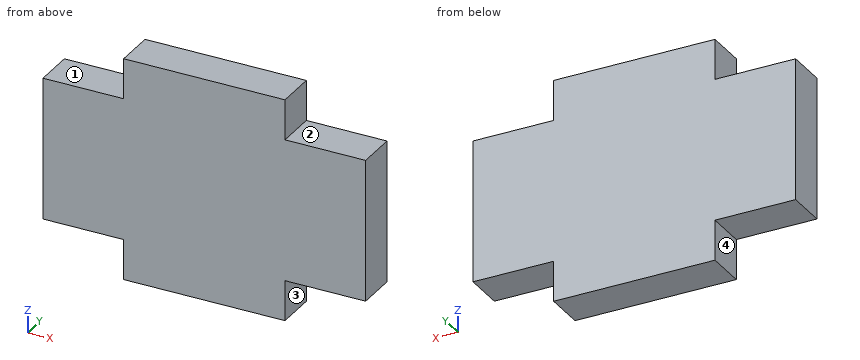
```python
from build123d import *

# Parameters (mm, degrees)
SKETCH1_W           = 12.7
SKETCH1_H           = 3.175
SKETCH1_W_2         = 6.35
BOSS_EXTRUDE1_DEPTH = 3.175


with BuildPart() as part:
    # Sketch1 → Boss-Extrude1 (new body)
    with BuildSketch(Plane(origin=(0, 0, 0), x_dir=(1, 0, 0), z_dir=(0, 1, 0))):
        Polygon((0, 11.176), (0, 0), (6.35, 0), (19.05, 0), (25.4, 0), (25.4, 11.176), (19.05, 11.176), (12.7, 11.176), (6.35, 11.176), align=None)
        with Locations((12.7, -1.5875)):
            Rectangle(SKETCH1_W, SKETCH1_H)
        with Locations((15.875, 12.7635)):
            Rectangle(SKETCH1_W_2, SKETCH1_H)
        with Locations((9.525, 12.7635)):
            Rectangle(SKETCH1_W_2, SKETCH1_H)
    extrude(amount=BOSS_EXTRUDE1_DEPTH)


solid = part.part
```
Geometry check sheet. Reference: the model listing, model coordinates, mm. Face numbers are marked on the shaded views. A direction names the side the tool comes from. Round coordinates to 2 decimals unless told otherwise and drop trailing zeros. Loops run counter-clockwise (first coordinate to the right, second up) from the corner with the lowest first, then second, coordinate; pieces in that order, holes last. Notation, with made-up numbers: (17.25, -22.75) - (41.25, -22.75) arc R29 cw to (41.25, 4.25) - close; hole circle Ø7 at (31.25, 16). An arc over 180 degrees is marked (long way). Write each question's results on one line, items separated by ' | '. Start each with the question number.
Q1. Cross-section at C-C on z = 2. Enter the section's corners in (x, y) (3 decimals), and give its area (3 significant figures).
Q2. Cross-section at A-A on y = 0.5. Enter the section's corners in (x, z) (3 decimals).
Q3. Thickness scan on line 1 (Z direction, x = 5.5, y = 0.4); line 2 (X direction, y = 2.7, z = -12.75). Record the ranges inside material, lowest first. Write a range as [from, to].
Q4. Gauge pin test, flat ends, axial feed: P1, Ø1, axis at y = 2, z = 1.5, coming from the +X side; P2, Ø1, axis at x = 23.5, y = 2, coming from the -Z side; P3, Ø1.6, axis at x = 2.5, y = 2, coming from the +Z side. Record the tip position at first contact, or that the pin passes through.
Q5. Cross-section at B-B on x = 2.5. Enter the section's corners in (y, z) (3 decimals), and give its area (3 significant figures).
Q6. Access from +Z, -Z, +X, -X, +Y, -Y to the whole of each face (thin tool, end or side, straight path). Record for the marked faces 1, 2, 3 and 4.
Answers below:
1) outline: (6.35, 0) - (19.05, 0) - (19.05, 3.175) - (6.35, 3.175) - close | area: 40.3 mm²
2) outline: (0, -11.176) - (6.35, -11.176) - (6.35, -14.351) - (19.05, -14.351) - (19.05, -11.176) - (25.4, -11.176) - (25.4, 0) - (19.05, 0) - (19.05, 3.175) - (6.35, 3.175) - (6.35, 0) - (0, 0) - close
3) line 1: z = [-11.18, 0] | line 2: x = [6.35, 19.05]
4) P1: stops at x = 19.05 | P2: stops at z = -11.18 | P3: stops at z = 0
5) outline: (0, -11.176) - (3.175, -11.176) - (3.175, 0) - (0, 0) - close | area: 35.5 mm²
6) face 1: +Z, -X, +Y, -Y | face 2: +Z, +X, +Y, -Y | face 3: -Z, +X, +Y, -Y | face 4: -Z, -X, +Y, -Y
